Can you work these out from the drawing? Everything is in mm from the part's minimum corner. Round coordinates to 2 decimals unless told otherwise and drop trailing zeros. Write each loop counter-clockwise with the first axis right and the second up, starting at its lowest first coordinate (ties: lowest second). Pieces come first, ordered by that corner, then holes. Notation, with made-up numbers: M 86.25,19 L 127.25,19 A16 cw 127.25,50 Z; hole C 3,-3.75 d4. An arc over 180 degrees is marked long. Use one line per item in the form item = value. Start each with the question number.
Q1. We'd pull the mould along X, two halves only. Please class the marked faces 1, 2 and 3: +X half, -X half, draft (parallel to the pull), parting line (faces both ways), or undercut.
Q2. I want a section at A-A on y = 20.5. List the corners of the cut face in (x, z) for me, and give its area (3 significant figures).
Q3. I want a section at D-D on z = 5.75. List the corners of the cut face in (x, y) for me.
Q4. I want a section at B-B on x = 20.5. List the corners of the cut face in (y, z) for me.
Q5. I need wall thicknesses on line 1 along Y through (x, z) = (20.5, 2.5); line 2 along Y through (x, z) = (20.5, 5.25); line 3 along Z through (x, y) = (28, 36). Which ranges of each line are inside material? Lowest first, please. Write a range as from..to.
Q6. I want a section at C-C on z = 1.75. List the corners of the cut face in (x, y) for me, and give its area (3 significant figures).
Q7. I'm going to push flat-ended pins straight in: pin 1 Ø1.5 at (y, z) = (35.5, 4.5) entering from -X; pin 2 Ø1.7 at (x, z) = (37.5, 2) entering from +Y (1 decimal). Where does each tip first touch, or does it pass through?
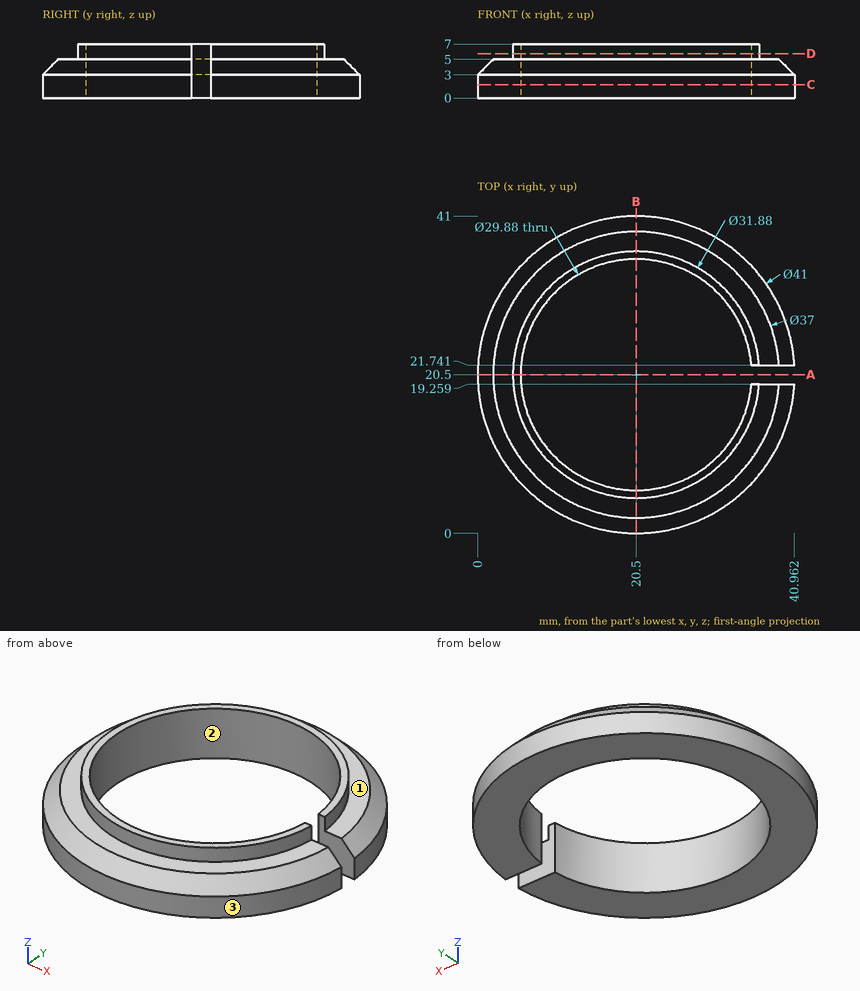
Reported:
q1.face_1 = draft
q1.face_2 = undercut
q1.face_3 = parting line
q2.outline = M 0,0 L 5.56,0 L 5.56,7 L 4.56,7 L 4.56,5 L 2,5 L 0,3 Z
q2.area = 27.8 mm^2
q3.outline = M 35.39,19.26 A14.94 cw long 35.39,21.74 L 36.39,21.74 A15.94 ccw long 36.39,19.26 Z
q4.outline = M 0,0 L 5.56,0 L 5.56,7 L 4.56,7 L 4.56,5 L 2,5 L 0,3 Z; M 35.44,0 L 41,0 L 41,3 L 39,5 L 36.44,5 L 36.44,7 L 35.44,7 Z
q5.line_1 = 0..5.56, 35.44..41
q5.line_2 = 4.56..5.56, 35.44..36.44
q5.line_3 = 0..5
q6.outline = M 35.39,19.26 A14.94 cw long 35.39,21.74 L 40.96,21.74 A20.5 ccw long 40.96,19.26 Z
q6.area = 605 mm^2
q7.pin_1 = 7.37
q7.pin_2 = 33.1
